Model file for the job. Use its own axes, mm. A direction names the side the tool comes from. Coordinates: 2 decimals unless noted, no trailing zeros. Order: outer loops, then holes, each group sorted by start corner. A loop starts at its lowest first (then second) coordinate and runs counter-clockwise, first axis right, second up. Notation, with made-up numbers: (24, -29.75) -> (43, -29.75) arc R23 ccw to (43, -5.75) -> close; hole circle Ø8 at (-23, 12). An arc over 180 degrees is marked (long way). Use CSV: the item, a comma, the result in double quotes. Start each with the question number.
(1) Tool access for faces 3 (the flat face through (-595, 96, 1089)), 4 (the flat face through (-8, -119, 1020)), 5 (the flat face through (-593, 148, 739)): list every direction of +Z, -Z, +X, -X, +Y, -Y with a clear straight run to the whole face (end or side of a thin tool).
(2) Pin check, flat tips, straight feed: pin 1 Ø6 at (x, y) = (458, 59.5) entering from +Z; pin 2 Ø24 at (x, z) = (82, 742.5) entering from -Y; pin 3 Ø24 at (y, z) = (-202.5, 754) entering from +X. Stop position of each tip, or through.
(3) Cut at B-B on y = 54.5. Give the number of separate pieces and of enclosed holes in the cut face, plus the area to 3 significant figures.
(4) Probe L1, parallel to Y at x = -309, z = 1116; L2, parallel to Y at x = 18, z = 775.5; L3, parallel to Z at x = 219.5, y = 79.5. List the from-to ranges inside material, lowest first.
(5) Cut at A-A on z = 1541. Write the cut outline in (x, y), plus the area to 3 significant figures.
(6) Pull direction Z, two halves, no side cores. Call faces 1 (the flat face through (8.4, 182.52, 2164.51)), 2 (the flat face through (8, -213, 1089)): pulls with the +Z half, pulls with the -Z half, needs draft (parallel to the pull), parting line crosses it, or undercut.
```python
from build123d import *

# Parameters (mm, degrees)
F2_W      = 1100
F2_H      = 620
F3_DEPTH  = 150
F4_W      = 1200
F4_H      = 720
F5_DEPTH  = 550
F6_W      = 1200
F6_H      = 40
F7_DEPTH  = 700
F9_W      = 1200
F9_H      = 440
F10_DEPTH = 30
F11_W     = 1200
F11_H     = 160
F12_DEPTH = 30
F13_R     = 80
F14_R     = 85
F15_R     = 50
F16_R     = 50
F18_DEPTH = 80
F20_DEPTH = 80
F23_DEPTH = 1200
F25_DEPTH = 5
F27_DEPTH = 5
F29_DEPTH = 5
F31_DEPTH = 5
F32_R     = 15
F33_DEPTH = 794.9063180602
F35_DEPTH = 150


with BuildPart() as f3:
    # F2 (on Top) → F3 (new body, through all)
    with BuildSketch(Plane.XY):
        Rectangle(F2_W, F2_H)
    extrude(amount=F3_DEPTH)

    # F4 (on face) → F5 (join, through all)
    with BuildSketch(Plane.XY.offset(150)):
        Rectangle(F4_W, F4_H)
    extrude(amount=F5_DEPTH)

    # F6 (on face) → F7 (join, through all)
    with BuildSketch(Plane.XY.offset(700)):
        Rectangle(F6_W, F6_H)
    extrude(amount=F7_DEPTH)

    # F9 (on plane+point) → F10 (join, through all)
    with BuildSketch(Plane.XY.offset(1020)):
        Rectangle(F9_W, F9_H)
    extrude(amount=F10_DEPTH)

    # F11 (on face) → F12 (join, through all)
    with BuildSketch(Plane.XY.offset(1400)):
        Rectangle(F11_W, F11_H)
    extrude(amount=-F12_DEPTH)

    # F13
    f13_edges = [f3.edges().sort_by_distance(p)[0] for p in [
        (600, -360, 425),
        (-600, -360, 425),
        (600, 360, 425),
        (-600, 360, 425),
    ]]
    fillet(f13_edges, radius=F13_R)

    # F14
    f14_edges = [f3.edges().sort_by_distance(p)[0] for p in [
        (-550, 310, 75),
        (-550, -310, 75),
        (550, -310, 75),
        (550, 310, 75),
    ]]
    fillet(f14_edges, radius=F14_R)

    # F15
    f15_edges = [f3.edges().sort_by_distance(p)[0] for p in [
        (600, 220, 1035),
        (-600, 220, 1035),
        (-600, -220, 1035),
        (600, -220, 1035),
    ]]
    fillet(f15_edges, radius=F15_R)

    # F16
    f16_edges = [f3.edges().sort_by_distance(p)[0] for p in [
        (600, -80, 1385),
        (600, 80, 1385),
        (-600, -80, 1385),
        (-600, 80, 1385),
    ]]
    fillet(f16_edges, radius=F16_R)

    # F17 (on face) → F18 (join)
    with BuildSketch(Plane.XY.offset(700)):
        with BuildLine():
            ThreePointArc((-520, 355), (-573.033008589, 333.033008589), (-595, 280))
            Line((-595, 280), (-595, -280))
            ThreePointArc((-595, -280), (-573.033008589, -333.033008589), (-520, -355))
            Line((-520, -355), (520, -355))
            ThreePointArc((520, -355), (573.033008589, -333.033008589), (595, -280))
            Line((595, -280), (595, 280))
            ThreePointArc((595, 280), (573.033008589, 333.033008589), (520, 355))
            Line((520, 355), (-520, 355))
        make_face()
        with BuildLine():
            ThreePointArc((593, -280), (571.6187950266, -331.6187950266), (520, -353))
            Line((520, -353), (-520, -353))
            ThreePointArc((-520, -353), (-571.6187950266, -331.6187950266), (-593, -280))
            Line((-593, -280), (-593, 280))
            ThreePointArc((-593, 280), (-571.6187950266, 331.6187950266), (-520, 353))
            Line((-520, 353), (520, 353))
            ThreePointArc((520, 353), (571.6187950266, 331.6187950266), (593, 280))
            Line((593, 280), (593, -280))
        make_face(mode=Mode.SUBTRACT)
    extrude(amount=F18_DEPTH)

    # F19 (on face) → F20 (join)
    with BuildSketch(Plane.XY.offset(1050)):
        with BuildLine():
            ThreePointArc((-550, 215), (-581.8198051534, 201.8198051534), (-595, 170))
            Line((-595, 170), (-595, 15))
            Line((-595, 15), (-595, -15))
            Line((-595, -15), (-595, -170))
            ThreePointArc((-595, -170), (-581.8198051534, -201.8198051534), (-550, -215))
            Line((-550, -215), (550, -215))
            ThreePointArc((550, -215), (581.8198051534, -201.8198051534), (595, -170))
            Line((595, -170), (595, -15))
            Line((595, -15), (595, 15))
            Line((595, 15), (595, 170))
            ThreePointArc((595, 170), (581.8198051534, 201.8198051534), (550, 215))
            Line((550, 215), (-550, 215))
        make_face()
        with BuildLine():
            Line((593, 170), (593, 15))
            Line((593, 15), (593, -15))
            Line((593, -15), (593, -170))
            ThreePointArc((593, -170), (580.405591591, -200.405591591), (550, -213))
            Line((550, -213), (-550, -213))
            ThreePointArc((-550, -213), (-580.405591591, -200.405591591), (-593, -170))
            Line((-593, -170), (-593, -15))
            Line((-593, -15), (-593, 15))
            Line((-593, 15), (-593, 170))
            ThreePointArc((-593, 170), (-580.405591591, 200.405591591), (-550, 213))
            Line((-550, 213), (550, 213))
            ThreePointArc((550, 213), (580.405591591, 200.405591591), (593, 170))
        make_face(mode=Mode.SUBTRACT)
    extrude(amount=F20_DEPTH)



with BuildPart() as f23:
    # F22 (on face) → F23 (new body, through all)
    with BuildSketch(Plane.YZ.offset(600)):
        Polygon((360, 2130), (0, 2200), (-360, 2130), (-359.2919978771, 2125.0439851397), (0, 2194.9063180602), (359.2919978771, 2125.0439851397), align=None)
    extrude(amount=-F23_DEPTH)

    # F24 (on face) → F25 (join)
    with BuildSketch(Plane.XZ.offset(360)):
        with BuildLine():
            Line((600, 2130), (-600, 2130))
            Line((-600, 2130), (-600, 1990))
            ThreePointArc((-600, 1990), (-540, 1930), (-480, 1990))
            ThreePointArc((-480, 1990), (-420, 1930), (-360, 1990))
            ThreePointArc((-360, 1990), (-300, 1930), (-240, 1990))
            ThreePointArc((-240, 1990), (-180, 1930), (-120, 1990))
            ThreePointArc((-120, 1990), (-60, 1930), (0, 1990))
            ThreePointArc((0, 1990), (60, 1930), (120, 1990))
            ThreePointArc((120, 1990), (180, 1930), (240, 1990))
            ThreePointArc((240, 1990), (300, 1930), (360, 1990))
            ThreePointArc((360, 1990), (420, 1930), (480, 1990))
            ThreePointArc((480, 1990), (540, 1930), (600, 1990))
            Line((600, 1990), (600, 2130))
        make_face()
    extrude(amount=-F25_DEPTH)

    # F26 (on face) → F27 (join)
    with BuildSketch(Plane(origin=(0, 360, 0), x_dir=(-1, 0, 0), z_dir=(0, 1, 0))):
        with BuildLine():
            Line((600, 1990), (600, 2130))
            Line((600, 2130), (-600, 2130))
            Line((-600, 2130), (-600, 1990))
            ThreePointArc((-600, 1990), (-540, 1930), (-480, 1990))
            ThreePointArc((-480, 1990), (-420, 1930), (-360, 1990))
            ThreePointArc((-360, 1990), (-300, 1930), (-240, 1990))
            ThreePointArc((-240, 1990), (-180, 1930), (-120, 1990))
            ThreePointArc((-120, 1990), (-60, 1930), (0, 1990))
            ThreePointArc((0, 1990), (60, 1930), (120, 1990))
            ThreePointArc((120, 1990), (180, 1930), (240, 1990))
            ThreePointArc((240, 1990), (300, 1930), (360, 1990))
            ThreePointArc((360, 1990), (420, 1930), (480, 1990))
            ThreePointArc((480, 1990), (540, 1930), (600, 1990))
        make_face()
    extrude(amount=-F27_DEPTH)

    # F28 (on face) → F29 (join)
    with BuildSketch(Plane.YZ.offset(600)):
        with BuildLine():
            Line((360, 2130), (0, 2200))
            Line((0, 2200), (-360, 2130))
            Line((-360, 2130), (-360, 1990))
            ThreePointArc((-360, 1990), (-300, 1930), (-240, 1990))
            ThreePointArc((-240, 1990), (-180, 1930), (-120, 1990))
            ThreePointArc((-120, 1990), (-60, 1930), (0, 1990))
            ThreePointArc((0, 1990), (60, 1930), (120, 1990))
            ThreePointArc((120, 1990), (180, 1930), (240, 1990))
            ThreePointArc((240, 1990), (300, 1930), (360, 1990))
            Line((360, 1990), (360, 2130))
        make_face()
    extrude(amount=-F29_DEPTH)

    # F30 (on face) → F31 (join)
    with BuildSketch(Plane(origin=(-600, 0, 0), x_dir=(0, -1, 0), z_dir=(-1, 0, 0))):
        with BuildLine():
            Line((-360, 2130), (-360, 1990))
            ThreePointArc((-360, 1990), (-300, 1930), (-240, 1990))
            ThreePointArc((-240, 1990), (-180, 1930), (-120, 1990))
            ThreePointArc((-120, 1990), (-60, 1930), (0, 1990))
            ThreePointArc((0, 1990), (60, 1930), (120, 1990))
            ThreePointArc((120, 1990), (180, 1930), (240, 1990))
            ThreePointArc((240, 1990), (300, 1930), (360, 1990))
            Line((360, 1990), (360, 2130))
            Line((360, 2130), (0, 2200))
            Line((0, 2200), (-360, 2130))
        make_face()
    extrude(amount=-F31_DEPTH)


with BuildPart() as f3_1:
    add(f3.part)

    add(f23.part)  # F33 merges F23
    # F32 (on face) → F33 (join, through all)
    with BuildSketch(Plane.XY.offset(1400)):
        with Locations((-520, 0)):
            Circle(F32_R)
        with Locations((520, 0)):
            Circle(F32_R)
    extrude(amount=F33_DEPTH)

    # F34 (on face) → F35 (join, through all)
    with BuildSketch(Plane(origin=(0, 0, 150), x_dir=(1, 0, 0), z_dir=(0, 0, -1))):
        with BuildLine():
            Line((520, 360), (-520, 360))
            ThreePointArc((-520, 360), (-576.5685424949, 336.5685424949), (-600, 280))
            Line((-600, 280), (-600, -280))
            ThreePointArc((-600, -280), (-576.5685424949, -336.5685424949), (-520, -360))
            Line((-520, -360), (520, -360))
            ThreePointArc((520, -360), (576.5685424949, -336.5685424949), (600, -280))
            Line((600, -280), (600, 280))
            ThreePointArc((600, 280), (576.5685424949, 336.5685424949), (520, 360))
        make_face()
    extrude(amount=F35_DEPTH)


solid = f3_1.part
```
Outcome:
1,face 3,"-X, +Y"
1,face 4,"+X, -X, -Y"
1,face 5,"none"
2,pin 1,"z = 2189.01"
2,pin 2,"y = -355"
2,pin 3,"x = 595"
3,separate pieces,"4"
3,enclosed holes,"0"
3,area,"921,000 mm2"
4,L1,"-215 to -213, -20 to 20, 213 to 215"
4,L2,"-355 to -353, -20 to 20, 353 to 355"
4,L3,"0 to 700, 1020 to 1050, 1370 to 1400, 2179.45 to 2184.54"
5,outline,"circle Ø30 at (-520, 0); circle Ø30 at (520, 0)"
5,area,"1,410 mm2"
6,face 1,"pulls with the +Z half"
6,face 2,"undercut"
